```python
from build123d import *

# Parameters (mm, degrees)
F2_DEPTH = 25.4


with BuildPart() as f2:
    # F1 (on Front) → F2 (new body)
    with BuildSketch(Plane.XZ):
        with BuildLine():
            Line((83.1839653551, -92.7227025355), (93.3241924209, -51.3479548737))
            add(Edge.make_bspline(
                [(93.3241924209, -51.3479548737), (0, 95.9786721212), (-93.3241924209, -51.3479548737)],
                knots=[0.3102753039, 0.3102753039, 0.3102753039, 2.8313173497, 2.8313173497, 2.8313173497], degree=2, weights=[1, 0.3053208061, 1]))
            Line((-93.3241924209, -51.3479548737), (-83.1839653551, -92.7227025355))
            Line((-83.1839653551, -92.7227025355), (83.1839653551, -92.7227025355))
        make_face()
        Polygon((-66.6030276888, -72.0353287046), (-53.9340679584, -59.3353666377), (47.827086872, -59.3353666377), (53.9340679584, -59.3353666377), (66.6030276888, -72.0353287046), (53.9030656219, -84.704288435), (47.8580892086, -84.704288435), (-53.9030656219, -84.704288435), align=None, mode=Mode.SUBTRACT)
    extrude(amount=F2_DEPTH)


solid = f2.part
```
Work out the finished part from the listing and answer in its coordinate system (mm). A direction names the side the tool comes from. Give positions to 0.01 mm unless a question says otherwise; leave off trailing zeros. Loops run counter-clockwise (first coordinate to the right, second up) from the corner with the lowest first, then second, coordinate; pieces in that order, holes last. Notation, with made-up numbers: (-21, 62) - (-6, 62) arc R18 ccw to (-6, 82) - close; hole circle Ø11 at (38.5, 29.25). An arc over 180 degrees is marked (long way). One line per question, with ' | ' between items.
(1) The mould has two halves that part along Z. Classify faces 1 (the face through (-60.357, -12.522, -65.774)), 2 (the face through (0, 0, -47)), 3 (the face through (88.183, -12.522, -72.325)): +Z half, -Z half, draft (parallel to the pull), parting line (faces both ways), or undercut.
Recorded:
face 1: undercut | face 2: draft | face 3: -Z half
(2) The part is cut by section B-B (z = -82.5). Write down the section's boundary in (x, y).
Recorded:
outline: (-85.69, -25.4) - (-56.11, -25.4) - (-56.11, 0) - (-85.69, 0) - close; (56.11, -25.4) - (85.69, -25.4) - (85.69, 0) - (56.11, 0) - close
(3) Straight lines are drawn through the part: probe 1 along Z at (x, y) = (2.5, -17.25); probe 2 along Z at (x, y) = (-32, -23.5); probe 3 along X at (y, z) = (-14, -77). For each, find the intervals that lie inside material, in ascending order.
Recorded:
probe 1: z = -92.72 to -84.7, -59.34 to -16.9 | probe 2: z = -92.72 to -84.7, -59.34 to -19.61 | probe 3: x = -87.04 to -61.63, 61.63 to 87.04
(4) A tool of negligible diameter and unlimited length cuts with its end or side. For faces 4 (the face through (60.342, -12.522, -78.281)), 5 (the face through (-1, -13, -92.723)), from which of +Z, -Z, +X, -X, +Y, -Y can it reach the whole face along a straight path? Write none if from no direction.
Recorded:
face 4: +Y, -Y | face 5: -Z, +X, -X, +Y, -Y
(5) The part is cut by section A-A (z = -62). Write down the section's boundary in (x, y), then the cut area to 3 significant figures.
Recorded:
outline: (-90.71, -25.4) - (-56.59, -25.4) - (-56.59, 0) - (-90.71, 0) - close; (56.59, -25.4) - (90.71, -25.4) - (90.71, 0) - (56.59, 0) - close | area: 1,730 mm²
(6) Each of these flat-tipped pins is pushed along its axis until it touches: pin 1 Ø3 at (y, z) = (-10.5, -77.5) entering from -X; pin 2 Ø12 at (y, z) = (-3.5, -28.5) entering from -X; pin 3 Ø5 at (y, z) = (-4, -75.5) entering from -X. Where does it stop, or does it pass through?
Recorded:
pin 1: stops at x = -87.28 | pin 2: stops at x = -74.9 | pin 3: stops at x = -88.02
